```python
from build123d import *

# Parameters (mm, degrees)
F1_DEPTH = 1.5
F2_R     = 1.5
F3_DEPTH = 25


# Not quite as in the source:
# - the dataset's text gives a spline's control points without its knots; the knots are read off the source's solid


with BuildPart() as f1:
    # F0 (on Top) → F1 (new body, symmetric)
    with BuildSketch(Plane.XY):
        with BuildLine():
            add(Edge.make_bspline(
                [(-7.2290541015, -0.5527675977), (-3.9967772573, -0.8917449116), (-3.2988634653, -2.0894490401), (-1.0464995032, -2.9017509308)],
                knots=[0, 0, 0, 0, 6.6137511338, 6.6137511338, 6.6137511338, 6.6137511338], degree=3))
            ThreePointArc((-1.0464995032, -2.9017509308), (3.0587935975, -0.3988751709), (-0.2673646533, 3.0730824617))
            add(Edge.make_bspline(
                [(-3.0769753559, 2.4563793473), (-1.7409748989, 2.5984151431), (-1.6058379576, 2.9566324623), (-0.2673646533, 3.0730824617)],
                knots=[0, 0, 0, 0, 2.876497007, 2.876497007, 2.876497007, 2.876497007], degree=3))
            add(Edge.make_bspline(
                [(-3.0769753559, 2.4563793473), (-5.7816746579, 2.1906947352), (-11.4426782467, 2.6135423344), (-17.8801982674, 5.2791288997), (-21.4653904829, 7.5502048837), (-22.1168282691, 7.9895307861)],
                knots=[0.005973262, 0.005973262, 0.005973262, 0.005973262, 0.125, 0.25, 0.277850749, 0.277850749, 0.277850749, 0.277850749], degree=3))
            Line((-22.1168282691, 7.9895307861), (-23.0633222923, 7.3125738031))
            Line((-23.0633222923, 7.3125738031), (-54.4799332581, 61.7749325905))
            ThreePointArc((-54.4799332581, 61.7749325905), (-55.1628772285, 61.9582016093), (-55.3461462473, 61.2752576388))
            Line((-55.3461462473, 61.2752576388), (-23.8805872256, 6.7280448046))
            Line((-23.8805872256, 6.7280448046), (-24.6317860127, 6.1907680209))
            add(Edge.make_bspline(
                [(-7.2290541015, -0.5527675977), (-8.7909293011, -0.4393198693), (-13.6136774425, 0.3217510425), (-19.4562298082, 2.7561257866), (-23.6206363974, 5.4709704249), (-24.6317860127, 6.1907680209)],
                knots=[0.064829406, 0.064829406, 0.064829406, 0.064829406, 0.125, 0.25, 0.290542228, 0.290542228, 0.290542228, 0.290542228], degree=3))
        make_face()
    extrude(amount=F1_DEPTH, both=True)

    # F2 (on face) → F3 (cut)
    with BuildSketch(Plane(origin=(0, 0, -1.5), x_dir=(1, 0, 0), z_dir=(0, 0, -1))):
        Circle(F2_R)
    extrude(amount=-F3_DEPTH, mode=Mode.SUBTRACT)


solid = f1.part
```
Can you work these out from the model? Positions are in its coordinate system, mm. Round coordinates to 2 decimals unless told otherwise and drop trailing zeros. Loops run counter-clockwise (first coordinate to the right, second up) from the corner with the lowest first, then second, coordinate; pieces in that order, holes last. Notation, with made-up numbers: (13, -25.75) -> (26, -25.75) arc R21 ccw to (26, 8.25) -> close; hole circle Ø2 at (85, 38.25). An arc over 180 degrees is marked (long way). Answer in a Markdown table with one row per item.
Item 1: If I drill on probe 1 along Y at (x, z) = (0, -0.3); probe 2 along Y at (x, z) = (-28.5, 1.15); probe 3 along X at (y, z) = (13.5, -0.8), over which ranges is the centre line in solid material (lowest first)?
Answer block:
| item | result |
|---|---|
| probe 1 | -3.08 to -1.5, 1.5 to 3.08 |
| probe 2 | 14.74 to 16.74 |
| probe 3 | -27.79 to -26.63 |
Item 2: Will these pins go through, and if not, where does the flat tip stop? P1, Ø1.8, axis at x = 0, y = 0, coming from the -Z side; P2, Ø1, axis at y = 35.5, z = -0.5, coming from the +X side.
Answer block:
| item | result |
|---|---|
| P1 | through |
| P2 | x = -39.03 |
Item 3: Suppose I cut it at B-B, the plane y = 52.5. List the corners of the cut face in (x, z) for me.
Answer block:
| item | result |
|---|---|
| outline | (-50.28, -1.5) -> (-49.13, -1.5) -> (-49.13, 1.5) -> (-50.28, 1.5) -> close |
Item 4: Suppose I cut it at A-A, the plane x = -36.5. List the corners of the cut face in (y, z) for me, plus the area to 3 significant figures.
Answer block:
| item | result |
|---|---|
| outline | (28.6, -1.5) -> (30.61, -1.5) -> (30.61, 1.5) -> (28.6, 1.5) -> close |
| area | 6.00 mm² |
Item 5: We'd pull the mould along X, two halves only. Please class faces 1 (the flat face through (-28, 15, -1.5)), 2 (the cylindrical face through (-1.5, -0.07, -0.02)), 3 (the flat face through (-39.83, 34.38, 0.02)): released by +X, released by -X, zero draft, split by the parting line, or undercut.
Answer block:
| item | result |
|---|---|
| face 1 | zero draft |
| face 2 | undercut |
| face 3 | released by -X |
